from build123d import *

# Parameters (mm, degrees)
SKETCH_3_R          = 2.825
CUT_EXTRUDE_2_DEPTH = 35
SKETCH_14_R         = 0.877374271
CUT_EXTRUDE_5_DEPTH = 12
SKETCH_16_W         = 5.008881277
SKETCH_16_H         = 1
EXTRUDE_2_DEPTH     = 30
SKETCH_19_W         = 0.959066555
SKETCH_19_H         = 0.511502163
EXTRUDE_3_DEPTH     = 30
SKETCH_24_W         = 24.30212029
SKETCH_24_H         = 4
CUT_EXTRUDE_8_DEPTH = 9
SKETCH_25_R         = 1.43
CUT_EXTRUDE_9_DEPTH = 22


with BuildPart() as part:
    # Sketch 1 → Revolve 1 (revolve)
    with BuildSketch(Plane.XY, mode=Mode.PRIVATE) as revolve_1_sk:
        Polygon((0, 0), (0, 22), (4.87, 22), (10.87, 12.418858447), (14.37, 12.418858447), (20.37, 22), (25.24, 22), (25.24, 12.418858447), (35.24, 12.418858447), (35.24, 0), align=None)
    revolve(revolve_1_sk.sketch.rotate(Axis((-743.15639781, 0, 0), (1, 0, 0)), 90), axis=Axis((-743.15639781, 0, 0), (1, 0, 0)))

    # Sketch 3 → Cut-Extrude 2 (cut)
    with BuildSketch(Plane(origin=(35.24, 0, 0), x_dir=(0, 0, -1), z_dir=(1, 0, 0))):
        Circle(SKETCH_3_R)
    extrude(amount=-CUT_EXTRUDE_2_DEPTH, mode=Mode.SUBTRACT)

    # Sketch 14 → Cut-Extrude 5 (cut)
    with BuildSketch(Plane.ZY):
        with Locations((-0.435299539, 17.00388826)):
            Circle(SKETCH_14_R)
    extrude(amount=-CUT_EXTRUDE_5_DEPTH, mode=Mode.SUBTRACT)

    # Sketch 16 → Extrude 2 (add)
    with BuildSketch(Plane(origin=(35.24, 0, 0), x_dir=(0, 0, -1), z_dir=(1, 0, 0))):
        with Locations((-0.105543204, 2.350977924)):
            Rectangle(SKETCH_16_W, SKETCH_16_H)
    extrude(amount=-EXTRUDE_2_DEPTH)

    # Sketch 19 → Extrude 3 (add)
    with BuildSketch(Plane(origin=(35.24, 0, 0), x_dir=(0, 0, -1), z_dir=(1, 0, 0))):
        with Locations((-0.084116996, 2.673942601)):
            Rectangle(SKETCH_19_W, SKETCH_19_H)
    extrude(amount=-EXTRUDE_3_DEPTH)

    # Sketch 24 → Cut-Extrude 8 (cut)
    with BuildSketch(Plane(origin=(35.24, 0, 0), x_dir=(0, 0, -1), z_dir=(1, 0, 0))):
        with Locations((0, 4.565108671)):
            Rectangle(SKETCH_24_W, SKETCH_24_H)
    extrude(amount=-CUT_EXTRUDE_8_DEPTH, mode=Mode.SUBTRACT)

    # Sketch 25 → Cut-Extrude 9 (cut)
    with BuildSketch(Plane(origin=(0, 22, 0), x_dir=(1, 0, 0), z_dir=(0, 1, 0))):
        with Locations(Location((29.956679037, 0, 0), (0, 0, 90))):
            Circle(SKETCH_25_R)
    extrude(amount=-CUT_EXTRUDE_9_DEPTH, mode=Mode.SUBTRACT)


solid = part.part
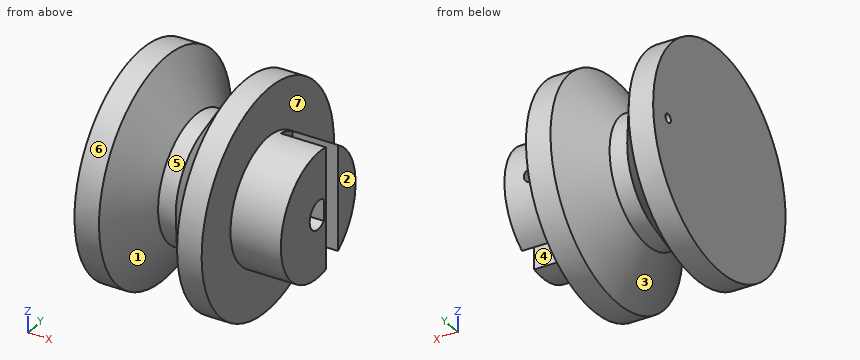
The model under review builds one solid part; all positions refer to its coordinate system, in mm. Face numbers are marked on the shaded views. A direction names the side the tool comes from. Round coordinates to 2 decimals unless told otherwise and drop trailing zeros. Order: outer loops, then holes, each group sorted by start corner. A loop starts at its lowest first (then second) coordinate and runs counter-clockwise, first axis right, second up. Notation, with made-up numbers: (75, -2) -> (112, -2) arc R25 cw to (112, 27) -> close; hole circle Ø2 at (59, 4.25). An arc over 180 degrees is marked (long way). Return JSON: item names as keys, results as strings.
1. The part is to be moulded in two halves that separate along X. For the marked faces 1, 2, 3 and 4, say which applies: +X half, -X half, draft (parallel to the pull), parting line (faces both ways), or undercut.
Answer block:
{"face 1": "undercut", "face 2": "+X half", "face 3": "undercut", "face 4": "draft"}
2. Insertion check: P1, Ø5, axis at x = 13, z = -10.5, coming from the +Y side; P2, Ø1.6, axis at y = 17, z = -0.44, coming from the -X side; P3, Ø3.5, axis at x = 21.5, z = 0.5, coming from the -Y side. Each pin has a flat end and moves straight along its axis. Give the tip position at first contact, or say it passes through.
Answer block:
{"P1": "stops at y = 10.13", "P2": "stops at x = 16.74", "P3": "stops at y = -22"}
3. For L1, parallel to X at y = 8, z = 0; L2, parallel to Y at x = 13, z = 0 (3 decimals); L3, parallel to X at y = -13, z = 0, list the stretches that pass through material, from the lowest coordinate up. Write a range as [from, to].
Answer block:
{"L1": "x = [0, 28.53], [31.39, 35.24]", "L2": "y = [-12.419, -2.825], [1.851, 12.419]", "L3": "x = [0, 10.51], [14.73, 25.24]"}
4. For the marked faces 5, 6 and 7, list the 3-axis set-ups (+Z, -Z, +X, -X, +Y, -Y) from which the entire face can be reached by the end or side of a thin tool; tool diameter is ignored.
Answer block:
{"face 5": "none", "face 6": "+X, -X", "face 7": "+X"}
5. Take a section at A-A (y = 0). Write out the cut boundary in (x, z) (3 decimals), then the cut area to 3 significant figures.
Answer block:
{"outline": "(0, -22) -> (4.87, -22) -> (10.87, -12.419) -> (14.37, -12.419) -> (20.37, -22) -> (25.24, -22) -> (25.24, -12.419) -> (35.24, -12.419) -> (35.24, -2.825) -> (0.24, -2.825) -> (0.24, 2.825) -> (35.24, 2.825) -> (35.24, 12.419) -> (25.24, 12.419) -> (25.24, 22) -> (20.37, 22) -> (14.37, 12.419) -> (10.87, 12.419) -> (4.87, 22) -> (0, 22) -> close", "area": "979 mm²"}
6. Take a section at B-B (x = 4). Write out the cut boundary in (y, z) (3 decimals), then the cut area to 3 significant figures.
Answer block:
{"outline": "circle Ø44 at (0, 0); hole circle Ø5.65 at (0, 0); hole circle Ø1.755 at (17.004, -0.435)", "area": "1,490 mm²"}
